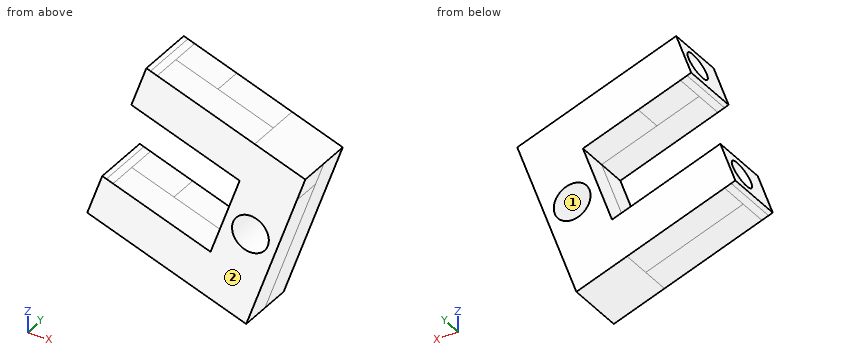
Autodesk Inventor part; units mm, degrees
ref_plane "YZ Plane" through (0, 0, 0) normal (1, 0, 0) x (0, 1, 0)
ref_plane "XZ Plane" through (0, 0, 0) normal (0, 1, 0) x (-1, 0, 0)
ref_plane "XY Plane" through (0, 0, 0) normal (0, 0, 1) x (1, 0, 0)
sketch "Sketch1" plane through (0, 0, 0) normal (0, 1, 0) x (-1, 0, 0)
  line L0 (6.5094, 9.5985) -> (7.4635, 6.913)
  line L1 (10.1521, -0.6544) -> (11.1062, -3.34)
  line L2 (-11.9694, 3.8348) -> (7.7922, 10.8558)
  line L3 (9.0875, 7.21) -> (-10.6741, 0.1891)
  line L4 (-8.1622, -6.8813) -> (11.5995, 0.1397)
  line L5 (12.8948, -3.5061) -> (-6.8669, -10.5271)
  line L6 (-6.8669, -10.5271) -> (-8.1622, -6.8813)
  line L7 (11.5995, 0.1397) -> (12.8948, -3.5061)
  line L8 (7.7922, 10.8558) -> (9.0875, 7.21)
  line L9 (-10.6741, 0.1891) -> (-11.9694, 3.8348)
  line L10 (6.9865, 8.2558) -> (-11.2395, 1.7804)
  line L11 (10.6292, -1.9972) -> (-7.5968, -8.4726)
  circle A0 centre (-12.8288, -4.5578) radius 1.5875
  line L12 (-12.8288, -4.5578) -> (-11.2395, 1.7804)
  line L13 (-7.5968, -8.4726) -> (-12.8288, -4.5578)
  line L14 (-11.2395, 1.7804) -> (-7.5968, -8.4726)
  line L15 (-6.8669, -10.5271) -> (-11.2395, -12.0806)
  line L16 (-11.2395, -12.0806) -> (-15.6121, 0.2269)
  line L17 (-15.6121, 0.2269) -> (-11.2395, 1.7804)
  line L18 (6.5094, 9.5985) -> (-11.7166, 3.1231)
  line L19 (7.4635, 6.913) -> (-10.7624, 0.4376)
  line L20 (10.1521, -0.6544) -> (-8.0739, -7.1298)
  line L21 (11.1062, -3.34) -> (-7.1197, -9.8154)
  line L22 (11.645, -4.8563) -> (9.3537, 1.5929)
  line L23 (-11.9694, 3.8348) -> (-16.342, 2.2813)
  line L24 (-16.342, 2.2813) -> (-15.6121, 0.2269)
  line L25 (-11.9694, 3.8348) -> (-11.2395, 1.7804)
  line L26 (6.9865, 8.2558) -> (-2.8266, 4.7693)
  line L27 (10.6292, -1.9972) -> (0.8161, -5.4836)
  line L28 (0.8161, -5.4836) -> (1.2932, -6.8264)
  line L29 (0.339, -4.1409) -> (0.8161, -5.4836)
  line L30 (-2.8266, 4.7693) -> (-2.3495, 3.4266)
  line L31 (-2.8266, 4.7693) -> (-3.3037, 6.1121)
  line L32 (-11.9694, 3.8348) -> (-3.5565, 6.8238)
  line L33 (-2.2612, 3.178) -> (-2.3495, 3.4266)
  line L34 (-2.2612, 3.178) -> (-10.6741, 0.1891)
  line L35 (0.339, -4.1409) -> (0.2507, -3.8923)
  line L36 (-8.1622, -6.8813) -> (0.2507, -3.8923)
  line L37 (1.2932, -6.8264) -> (1.546, -7.5381)
  line L38 (-6.8669, -10.5271) -> (1.546, -7.5381)
  line L39 (-6.8669, -10.5271) -> (-7.5968, -8.4726)
  line L40 (-3.3037, 6.1121) -> (-3.5565, 6.8238)
  point P0 (0, 0)
  dimension "d0" = 10.414
  dimension "d1" = 10.414
extrude "Extrusion1" add sketch "Sketch1" along normal blind 2.54 contours L31 L10 L9 L18 | L18 L9 L2 L40 | L30 L19 L9 L10 | L9 L17 L24 L23 | L33 L3 L9 L19 | L9 L14 L6 L13 A0 L12 | L12 A0 L16 L17 | L12 L13 A0 L16 | A0 L13 L12 | L4 L35 L20 L6 | L13 L6 L15 L16 A0 | L20 L29 L11 L6 | L11 L28 L21 L6 | L21 L37 L5 L6
sketch "Sketch2" plane through (0, 2.54, 0) normal (0, 1, 0) x (1, 0, 0)
  line L0 (11.2395, 12.0806) -> (-1.546, 7.5381)
  line L1 (-1.546, 7.5381) -> (2.092, 8.8306)
  line L2 (2.092, 8.8306) -> (3.3873, 5.1848)
  line L3 (-0.2507, 3.8923) -> (8.1622, 6.8813)
  line L4 (-0.2507, 3.8923) -> (3.3873, 5.1848)
  line L5 (-1.546, 7.5381) -> (-0.2507, 3.8923)
  line L6 (-0.2507, 3.8923) -> (-1.546, 7.5381)
  line L7 (2.2612, -3.178) -> (3.5565, -6.8238)
  line L8 (2.2612, -3.178) -> (3.5565, -6.8238)
  line L9 (3.5565, -6.8238) -> (7.1945, -5.5313)
  line L10 (3.5565, -6.8238) -> (16.342, -2.2813)
  line L11 (7.1945, -5.5313) -> (5.8992, -1.8855)
  line L12 (10.6741, -0.1891) -> (2.2612, -3.178)
  line L13 (2.2612, -3.178) -> (5.8992, -1.8855)
  point P0 (0, 0)
  dimension "d4" = 3.8608
  dimension "d5" = 3.8608
extrude "Extrusion2" add sketch "Sketch2" along normal blind 2.54
sketch "Sketch3" plane through (0, 2.54, 0) normal (0, 1, 0) x (1, 0, 0)
  line L0 (8.1622, 6.8813) -> (10.6741, -0.1891)
  line L1 (8.1622, 6.8813) -> (6.8669, 10.5271)
  line L2 (11.2395, 12.0806) -> (-1.546, 7.5381)
  line L3 (10.6615, -0.1534) -> (11.9694, -3.8348)
  line L4 (7.1945, -5.5313) -> (16.342, -2.2813)
  line L5 (6.8669, 10.5271) -> (2.092, 8.8306)
  line L6 (3.3873, 5.1848) -> (8.1622, 6.8813)
  line L7 (3.3873, 5.1848) -> (8.1622, 6.8813)
  line L8 (8.1622, 6.8813) -> (3.3873, 5.1848)
  line L9 (3.3873, 5.1848) -> (2.092, 8.8306)
  line L10 (2.092, 8.8306) -> (3.3873, 5.1848)
  line L11 (10.6741, -0.1891) -> (5.8992, -1.8855)
  line L12 (5.8992, -1.8855) -> (10.6741, -0.1891)
  line L13 (10.6741, -0.1891) -> (11.9694, -3.8348)
  line L14 (5.8992, -1.8855) -> (7.1945, -5.5313)
  line L15 (11.9694, -3.8348) -> (7.1945, -5.5313)
  line L16 (7.1945, -5.5313) -> (5.8992, -1.8855)
  point P0 (0, 0)
extrude "Extrusion3" add sketch "Sketch3" along normal blind 2.54
sketch "Sketch6" plane through (0, 2.54, 0) normal (0, 1, 0) x (1, 0, 0)
  line L0 (8.1622, 6.8813) -> (10.6741, -0.1891)
  line L1 (8.1622, 6.8813) -> (12.5348, 8.4348)
  line L2 (16.342, -2.2813) -> (11.2395, 12.0806)
  line L3 (10.6741, -0.1891) -> (15.0468, 1.3644)
  line L4 (15.0468, 1.3644) -> (12.8604, 0.5877)
  line L5 (10.3485, 7.658) -> (12.8604, 0.5877)
  line L6 (10.3485, 7.658) -> (9.0532, 11.3038)
  line L7 (11.2395, 12.0806) -> (-1.546, 7.5381)
  line L8 (12.8604, 0.5877) -> (14.1557, -3.0581)
  line L9 (11.9694, -3.8348) -> (16.342, -2.2813)
  circle A0 centre (11.6045, 4.1229) radius 1.4859
  point P0 (0, 0)
  dimension "d28" = 2.9718
hole "Hole3" at (11.6045, 2.54, -4.1229) direction (0, -1, 0) diameter 3.175 depth 7.62
sketch "Sketch7" plane through (0, 2.54, 0) normal (0, 1, 0) x (1, 0, 0)
  circle A0 centre (11.6045, 4.1229) radius 1.5875
  line L0 (10.6741, -0.1891) -> (11.9694, -3.8348)
  line L1 (11.9694, -3.8348) -> (16.342, -2.2813)
  line L2 (16.342, -2.2813) -> (11.2395, 12.0806)
  line L3 (11.2395, 12.0806) -> (6.8669, 10.5271)
  line L4 (6.8669, 10.5271) -> (8.1622, 6.8813)
  line L5 (8.1622, 6.8813) -> (10.6741, -0.1891)
  point P0 (0, 0)
extrude "Extrusion4" add sketch "Sketch7" along normal blind 2.54 contours A0 | L5 L4 L3 L2 L1 L0
sketch "Sketch8" plane through (11.6045, 2.54, -4.1229) normal (0, -1, 0) x (1, 0, 0)
  circle A0 centre (0, 0) radius 1.5875
  point P0 (-11.6045, 4.1229)
hole "Hole4" at (11.6045, 2.54, -4.1229) direction (0, 1, 0) diameter 3.175 depth 7.62
sketch "Sketch9" plane through (0, 0, 0) normal (0, -1, 0) x (1, 0, 0)
  line L0 (3.5565, 6.8238) -> (16.342, 2.2813)
  line L1 (10.6741, 0.1891) -> (2.2612, 3.178)
  line L2 (-0.2507, -3.8923) -> (8.1622, -6.8813)
  line L3 (11.2395, -12.0806) -> (-1.546, -7.5381)
  line L4 (3.5565, 6.8238) -> (16.342, 2.2813)
  line L5 (3.5565, 6.8238) -> (2.9821, 7.0279)
  line L6 (10.5107, 3.6362) -> (3.3304, 6.1873)
  line L7 (2.9821, 7.0279) -> (1.6868, 3.3821)
  line L8 (2.2612, 3.178) -> (3.5565, 6.8238)
  line L9 (1.6868, 3.3821) -> (2.2612, 3.178)
  line L10 (-1.546, -7.5381) -> (-0.2507, -3.8923)
  line L11 (-0.2507, -3.8923) -> (-0.8252, -3.6882)
  line L12 (-0.8252, -3.6882) -> (-2.1204, -7.334)
  line L13 (-2.1204, -7.334) -> (-1.4728, -7.5641)
  point P0 (0, 0)
  dimension "d45" = 0.6096
extrude "Extrusion5" add sketch "Sketch9" against normal blind 5.08
sketch "Sketch12" plane through (2.9821, 0, 7.0279) normal (-0.9422958, 0, 0.3347815) x (0.3347815, 0, 0.9422958)
  line L0 (0, 0) -> (-3.869, 0)
  line L1 (0, 0) -> (0, 5.08)
  line L2 (-3.869, 5.08) -> (0, 5.08)
  line L3 (-3.869, 0) -> (-3.869, 5.08)
  line L4 (-11.3724, 0) -> (-15.2414, 0)
  line L5 (-11.3724, 0) -> (-11.3724, 5.08)
  line L6 (-15.2414, 5.08) -> (-11.3724, 5.08)
  line L7 (-15.2414, 0) -> (-15.2414, 5.08)
  point P0 (-7.6207, 0)
extrude "Extrusion6" add sketch "Sketch12" along normal blind 0.381
sketch "Sketch15" plane through (2.6231, 0, 7.1554) normal (-0.9422958, 0, 0.3347815) x (0.3347815, 0, 0.9422958)
  line L0 (-11.3724, 5.08) -> (-15.2414, 5.08)
  line L1 (-15.2414, 5.08) -> (-15.2414, 0)
  point P0 (-7.6207, 0)
  point P1 (-13.3364, 3.175)
  dimension "d93" = 1.905
  dimension "d94" = 1.905
hole "Hole10" at (-1.8417, 3.175, -5.4114) direction (0.9422958, 0, -0.3347815) diameter 2.459 depth 8.7884
sketch "Sketch16" plane through (2.6231, 0, 7.1554) normal (-0.9422958, 0, 0.3347815) x (0.3347815, 0, 0.9422958)
  line L0 (0, 5.08) -> (-3.869, 5.08)
  line L1 (0, 0) -> (0, 5.08)
  point P0 (-7.6207, 0)
  point P1 (-1.905, 3.175)
  dimension "d102" = 1.905
  dimension "d103" = 1.905
hole "Hole11" at (1.9853, 3.175, 5.3604) direction (0.9422958, 0, -0.3347815) diameter 2.459 depth 8.7884
properties part number "fileholddub"
Geometry: final body of the model. Coordinates: model frame, mm. Face numbers are marked on the shaded views. Round coordinates to 2 decimals unless told otherwise and drop trailing zeros. Loops run counter-clockwise (first coordinate to the right, second up) from the corner with the lowest first, then second, coordinate; pieces in that order, holes last. Notation, with made-up numbers: M -15.5,6.5 L -1.5,6.5 A29 ccw -1.5,36.5 Z; hole C 51,3 d6. An arc over 180 degrees is marked long. Put each result on its own line as item: value. Start each with the question number.
(1) Section query B-B (x = 4). State how many separate pieces and enclosed holes the cut face has, then the cut area to 3 significant figures.
(2) Section query C-C (z = -0.5). Return loops of the section in (x, y), then the cut area to 3 significant figures.
(3) Draft query along Z for the marked faces 1 and 2. Return one class per face: +Z half, -Z half, draft (parallel to the pull), parting line (faces both ways), or undercut.
(4) Contact query for flat-ended pins moving along their axis: pin 1 Ø3 at (y, z) = (4.5, 3.5) entering from -X; pin 2 Ø3 at (x, y) = (6.5, 3.5) entering from -Z. Output: stop coordinate, or through.
(5) Material intervals for line 1 along Z through (x, y) = (6, 3.2); line 2 along Z through (x, y) = (5.5, 0.85); line 3 along Z through (x, y) = (7, 1.9), sorted ascending. Write a range as [from, to].
Findings below:
1. separate pieces: 2
1. enclosed holes: 2
1. area: 31.6 mm2
2. outline: M 10.43,0 L 15.35,0 L 15.35,5.08 L 10.43,5.08 Z
2. area: 25.0 mm2
3. face 1: undercut
3. face 2: draft
4. pin 1: stops at x = 1.33
4. pin 2: stops at z = -10.93
5. line 1: z = [-10.22, -9.5], [-6.89, -6.11], [1.85, 2.63], [5.24, 5.96]
5. line 2: z = [-10.04, -5.94], [2.03, 6.13]
5. line 3: z = [-10.57, -6.47], [1.49, 5.6]
